Input: part model. Units: mm. Frame: model coordinates. A direction names the side the tool comes from. Round coordinates to 2 decimals unless told otherwise and drop trailing zeros. Loops run counter-clockwise (first coordinate to the right, second up) from the corner with the lowest first, then second, coordinate; pieces in that order, holes last. Notation, with made-up numbers: (1.25, 19) - (11.25, 19) arc R21 ccw to (11.25, 38) - close; hole circle Ø11 at (-26.75, 20). An arc over 180 degrees is marked (long way). Write each question's results on one line, items separated by ' | '.
from build123d import *

# Parameters (mm, degrees)
ESQUISSE2_W             = 18
ESQUISSE2_H             = 4.5
ENL_V_MAT_EXTRU_1_DEPTH = 12.5
ESQUISSE3_W             = 18
ESQUISSE3_H             = 3
ENL_V_MAT_EXTRU_2_DEPTH = 12.5
ESQUISSE4_W             = 5
ESQUISSE4_H             = 36
CHANFREIN1_SIZE         = 0.5


with BuildPart() as part:
    # Esquisse1 → Base-Révolution (revolve)
    with BuildSketch(Plane.XY, mode=Mode.PRIVATE) as base_r_volution_sk:
        with BuildLine():
            Line((18, 0), (-18, 0))
            Line((-18, 0), (-18, 5))
            Line((-18, 5), (-8, 5))
            Line((-8, 5), (-8, 6))
            ThreePointArc((-8, 6), (0, 10), (8, 6))
            Line((8, 6), (8, 5))
            Line((8, 5), (18, 5))
            Line((18, 5), (18, 0))
        make_face()
    revolve(base_r_volution_sk.sketch.rotate(Axis((0, 0, 0), (-1, 0, 0)), 90), axis=Axis((0, 0, 0), (-1, 0, 0)))

    # Esquisse2 → Enlèv. mat.-Extru.1 (cut, symmetric)
    with BuildSketch(Plane.XY):
        with Locations((0, 8.75)):
            Rectangle(ESQUISSE2_W, ESQUISSE2_H)
        with Locations((0, -8.75)):
            Rectangle(ESQUISSE2_W, ESQUISSE2_H)
    extrude(amount=ENL_V_MAT_EXTRU_1_DEPTH, both=True, mode=Mode.SUBTRACT)

    # Esquisse3 → Enlèv. mat.-Extru.2 (cut, symmetric)
    with BuildSketch(Plane(origin=(0, 0, 0), x_dir=(1, 0, 0), z_dir=(0, 1, 0))):
        with Locations((0, 9.5)):
            Rectangle(ESQUISSE3_W, ESQUISSE3_H)
        with Locations((0, -9.5)):
            Rectangle(ESQUISSE3_W, ESQUISSE3_H)
    extrude(amount=ENL_V_MAT_EXTRU_2_DEPTH, both=True, mode=Mode.SUBTRACT)

    # Esquisse4 → Boss.-Révol.1 (revolve)
    with BuildSketch(Plane(origin=(0, 0, 0), x_dir=(1, 0, 0), z_dir=(0, 1, 0))):
        with Locations((2.5, 0)):
            Rectangle(ESQUISSE4_W, ESQUISSE4_H)
    revolve(axis=Axis((0, 0, 0), (0, 0, -1)))

    # Chanfrein1
    chanfrein1_edges = [part.edges().sort_by_distance(p)[0] for p in [
        (-18, 0, 5),
        (-5, 0, 8),
        (-5, 0, -18),
        (18, 0, 5),
        (-5, 0, 18),
    ]]
    chamfer(chanfrein1_edges, length=CHANFREIN1_SIZE)


solid = part.part
1. Section query D-D, the plane x = 10.5. Output: boundary loops of the cut face in (y, z), plus the area to 3 significant figures.
Answer:
outline: circle Ø10 at (0, 0) | area: 78.5 mm^2
2. Section query B-B, the plane z = 0. Output: boundary loops of the cut face in (x, y).
Answer:
outline: (-18, -4.5) - (-17.5, -5) - (-8, -5) - (-8, -6) arc R10 ccw to (-7.6, -6.5) - (7.6, -6.5) arc R10 ccw to (8, -6) - (8, -5) - (17.5, -5) - (18, -4.5) - (18, 4.5) - (17.5, 5) - (8, 5) - (8, 6) arc R10 ccw to (7.6, 6.5) - (-7.6, 6.5) arc R10 ccw to (-8, 6) - (-8, 5) - (-17.5, 5) - (-18, 4.5) - close
3. Set-up query: faces 1 (the flat face through (3, -5, 8)), 2 (the flat face through (-8, -4, -4)), 3 (the cylindrical face through (-1.08, 4.88, -12.82)), 4 (the flat face through (8, -4, 4)). Return all of +Z, -Z, +X, -X, +Y, -Y with unobstructed straight access to the full face (end or side cutting, diameter ignored); none if empty.
Answer:
face 1: +Z | face 2: -X | face 3: -Z | face 4: +X
4. Section query C-C, the plane x = 0. Output: boundary loops of the cut face in (y, z).
Answer:
outline: (-6.5, -7.6) arc R10 ccw to (-6, -8) - (-5, -8) - (-5, -17.5) - (-4.5, -18) - (4.5, -18) - (5, -17.5) - (5, -8) - (6, -8) arc R10 ccw to (6.5, -7.6) - (6.5, 7.6) arc R10 ccw to (6, 8) - (5.5, 8) - (5, 8.5) - (5, 17.5) - (4.5, 18) - (-4.5, 18) - (-5, 17.5) - (-5, 8.5) - (-5.5, 8) - (-6, 8) arc R10 ccw to (-6.5, 7.6) - close
5. Line query: line 1 (Y direction, x = 0, z = 10); line 2 (X direction, y = 4.5, z = -14.5); line 3 (X direction, y = -2.75, z = -12.5). Output: solid intervals per line, ascending. Write a range as [from, to].
Answer:
line 1: [-5, 5] | line 2: [-2.18, 2.18] | line 3: [-4.18, 4.18]
6. Contact query for flat-ended pins moving along their axis: pin 1 (6 mm diameter, centred on x = -12.5, y = -5, fed in from +Z); pin 2 (2 mm diameter, centred on y = 1.5, z = -5.5, fed in from +X); pin 3 (3 mm diameter, centred on x = 14, y = 0.5, fed in from -Z). Output: stop coordinate, or through.
Answer:
pin 1: z = 4.58 | pin 2: x = 17.8 | pin 3: z = -5
